For this review, take the finished solid that the model builds, in its own axes (mm). Give positions to 0.01 mm unless a question says otherwise; leave off trailing zeros. Loops run counter-clockwise (first coordinate to the right, second up) from the corner with the lowest first, then second, coordinate; pieces in that order, holes last. Notation, with made-up numbers: (-25.75, 84) -> (-13.75, 84) arc R19 ccw to (-13.75, 107) -> close; hole circle Ø6 at (44.25, 24). An arc over 180 degrees is marked (long way). Answer as CSV lines item,"result". Start each with the question number.
Item 1: Add section C-C on x = 0. State the section outline as (y, z) points, plus the area to 3 significant figures.
Item 2: Add section B-B on y = 40. State the section outline as (x, z) points, plus the area to 3 significant figures.
Item 3: For L1, parallel to Y at x = 0, z = 0.65; L2, parallel to Y at x = -4, z = 1.1; L3, parallel to X at y = 0.5, z = 0.25, list the stretches that pass through material, from the lowest coordinate up. Write a range as from..to.
Item 4: Add section A-A on z = 1.15. State the section outline as (x, y) points.
Item 5: Add section D-D on x = 11. State the section outline as (y, z) points.
```python
from build123d import *

# Parameters (mm, degrees)
F0_R     = 12.7
F0_R_2   = 5
F1_DEPTH = 2.032


with BuildPart() as f1:
    # F0 (on Top) → F1 (new body)
    with BuildSketch(Plane.XY):
        with BuildLine():
            Line((2, 50), (-2, 50))
            ThreePointArc((-2, 50), (-7.656854, 47.656854), (-10, 42))
            Line((-10, 42), (-10, 12.103305))
            ThreePointArc((-10, 12.103305), (0, -15.7), (10, 12.103305))
            Line((10, 12.103305), (10, 42))
            ThreePointArc((10, 42), (7.656854, 47.656854), (2, 50))
        make_face()
        Circle(F0_R, mode=Mode.SUBTRACT)
        with Locations((0, 40)):
            Circle(F0_R_2, mode=Mode.SUBTRACT)
    extrude(amount=F1_DEPTH)


solid = f1.part
```
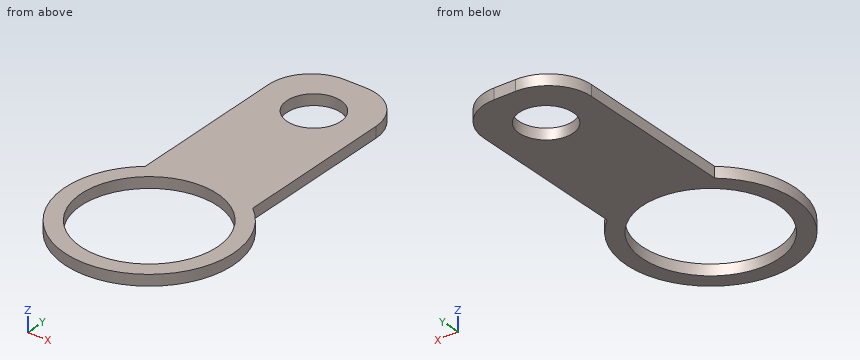
Computed values:
1,outline,"(-15.7, 0) -> (-12.7, 0) -> (-12.7, 2.03) -> (-15.7, 2.03) -> close; (12.7, 0) -> (35, 0) -> (35, 2.03) -> (12.7, 2.03) -> close; (45, 0) -> (50, 0) -> (50, 2.03) -> (45, 2.03) -> close"
1,area,"61.6 mm²"
2,outline,"(-10, 0) -> (-5, 0) -> (-5, 2.03) -> (-10, 2.03) -> close; (5, 0) -> (10, 0) -> (10, 2.03) -> (5, 2.03) -> close"
2,area,"20.3 mm²"
3,L1,"-15.7..-12.7, 12.7..35, 45..50"
3,L2,"-15.18..-12.05, 12.05..37, 43..49.75"
3,L3,"-15.69..-12.69, 12.69..15.69"
4,outline,"(-10, 12.1) arc R15.7 ccw (long way) to (10, 12.1) -> (10, 42) arc R8 ccw to (2, 50) -> (-2, 50) arc R8 ccw to (-10, 42) -> close; hole circle Ø25.4 at (0, 0); hole circle Ø10 at (0, 40)"
5,outline,"(-11.2, 0) -> (-6.35, 0) -> (-6.35, 2.03) -> (-11.2, 2.03) -> close; (6.35, 0) -> (11.2, 0) -> (11.2, 2.03) -> (6.35, 2.03) -> close"
